from build123d import *

# Parameters (mm, degrees)
SKETCH1_R           = 4
BOSS_EXTRUDE1_DEPTH = 111
CUT_EXTRUDE1_START  = -0.8
SKETCH2_R           = 4
SKETCH2_R_2         = 3.75
CUT_EXTRUDE1_DEPTH  = 0.8
SKETCH4_R           = 4
BOSS_EXTRUDE3_DEPTH = 0.85
BOSS_EXTRUDE4_START = 0.8
SKETCH3_R           = 3.75
BOSS_EXTRUDE4_DEPTH = 0.8
BOSS_EXTRUDE5_START = 1
SKETCH5_R           = 4
BOSS_EXTRUDE5_DEPTH = 1
SKETCH6_W           = 3
SKETCH6_H           = 3
CUT_EXTRUDE2_DEPTH  = 20


with BuildPart() as part:
    # Sketch1 → Boss-Extrude1 (new body)
    with BuildSketch(Plane(origin=(0, 0, 0), x_dir=(1, 0, 0), z_dir=(0, 1, 0))):
        with Locations(Location((0, 0, 0), (0, 0, 270))):
            Circle(SKETCH1_R)
    extrude(amount=BOSS_EXTRUDE1_DEPTH)

    # Sketch2 → Cut-Extrude1 (cut)
    with BuildSketch(Plane(origin=(0, 86, 0), x_dir=(1, 0, 0), z_dir=(0, 1, 0)).offset(CUT_EXTRUDE1_START)):
        with Locations(Location((0, 0, 0), (0, 0, 270))):
            Circle(SKETCH2_R)
        with Locations(Location((0, 0, 0), (0, 0, 270))):
            Circle(SKETCH2_R_2, mode=Mode.SUBTRACT)
    extrude(amount=CUT_EXTRUDE1_DEPTH, mode=Mode.SUBTRACT)

    # Sketch4 → Boss-Extrude3 (add)
    with BuildSketch(Plane(origin=(0, 111, 0), x_dir=(1, 0, 0), z_dir=(0, 1, 0))):
        with Locations(Location((0, 0, 0), (0, 0, 270))):
            Circle(SKETCH4_R)
    extrude(amount=BOSS_EXTRUDE3_DEPTH)

    # Sketch3 → Boss-Extrude4 (add)
    with BuildSketch(Plane(origin=(0, 0, 0), x_dir=(-1, 0, 0), z_dir=(0, -1, 0)).offset(BOSS_EXTRUDE4_START)):
        with Locations(Location((0, 0, 0), (0, 0, 270))):
            Circle(SKETCH3_R)
    extrude(amount=-BOSS_EXTRUDE4_DEPTH)

    # Sketch5 → Boss-Extrude5 (add)
    with BuildSketch(Plane.XZ.offset(0.8).offset(BOSS_EXTRUDE5_START)):
        with Locations(Location((0, 0, 0), (0, 0, 90))):
            Circle(SKETCH5_R)
    extrude(amount=-BOSS_EXTRUDE5_DEPTH)

    # Sketch6 → Cut-Extrude2 (cut)
    with BuildSketch(Plane(origin=(0, 111.85, 0), x_dir=(1, 0, 0), z_dir=(0, 1, 0))):
        with Locations((0, 4)):
            Rectangle(SKETCH6_W, SKETCH6_H)
    extrude(amount=-CUT_EXTRUDE2_DEPTH, mode=Mode.SUBTRACT)


solid = part.part
Source: CAD feature listing. Evaluate the final solid. Frame: model axes, mm. A direction names the side the tool comes from. Give positions to 0.01 mm unless a question says otherwise; leave off trailing zeros. Write each loop counter-clockwise with the first axis right and the second up, starting at its lowest first coordinate (ties: lowest second). Pieces come first, ordered by that corner, then holes. Notation, with made-up numbers: M 20.5,-37.75 L 41.5,-37.75 A29 ccw 41.5,-4.75 Z; hole C -27,45 d11. An arc over 180 degrees is marked long. Return JSON: item names as keys, results as strings. Group by question number.
1) Draft query along Y for faces 4 (the face through (0, -1.8, 0)), 5 (the face through (0.165, 85.594, -3.746)), 6 (the face through (0, 111.85, 0)), 7 (the face through (3.905, -1.307, -0.867)). Return one class per face: released by +Y, released by -Y, zero draft, split by the parting line, or undercut.
2) Cut plane C-C, the plane z = -1.25. Output: boundary loops of the cut face in (x, y), then the cut area to 3 significant figures.
3) First-contact query: pin 1 Ø1.5 at (x, y) = (-0.5, 30.5) entering from -Z; pin 2 Ø1 at (y, z) = (104, -3.5) entering from -X; pin 3 Ø0.8 at (x, z) = (-0.5, -3) entering from +Y; pin 4 Ø3.5 at (x, y) = (0, 101.5) entering from -Z. Flat tips, straight axial feed; report the tip coordinate or a pass-through.
4) Ray query, L1, parallel to Y at x = 3, z = -2.5; L2, parallel to Z at x = 0.25, y = 78; L3, parallel to X at y = 77.5, z = -3.5. Return the intervals inside material, ascending.
5) Cut plane B-B, the plane y = 58. Output: boundary loops of the cut face in (x, z), then the cut area to 3 significant figures.
6) Set-up query: faces 1 (the face through (-0.165, -0.406, -3.746)), 2 (the face through (-3.905, 42.004, -0.867)), 3 (the face through (0, 102, -2.5)). Return all of +Z, -Z, +X, -X, +Y, -Y with unobstructed straight access to the full face (end or side cutting, diameter ignored); none if empty.
7) Cut plane A-A, the plane x = 0. Output: boundary loops of the cut face in (y, z), then the cut area to 3 significant figures.
Data:
{
 "1": {"face 4": "released by -Y", "face 5": "undercut", "face 6": "released by +Y", "face 7": "zero draft"},
 "2": {"outline": "M -3.8,-1.8 L 3.8,-1.8 L 3.8,-0.8 L 3.54,-0.8 L 3.54,0 L 3.8,0 L 3.8,85.2 L 3.54,85.2 L 3.54,86 L 3.8,86 L 3.8,111.85 L -3.8,111.85 L -3.8,86 L -3.54,86 L -3.54,85.2 L -3.8,85.2 L -3.8,0 L -3.54,0 L -3.54,-0.8 L -3.8,-0.8 Z", "area": "863 mm²"},
 "3": {"pin 1": "stops at z = -4", "pin 2": "stops at x = -2.65", "pin 3": "stops at y = 91.85", "pin 4": "stops at z = -3.71"},
 "4": {"L1": "y = -1.8 to -0.8, 0 to 85.2, 86 to 111.85", "L2": "z = -3.99 to 3.99", "L3": "x = -1.94 to 1.94"},
 "5": {"outline": "C 0,0 d8", "area": "50.3 mm²"},
 "6": {"face 1": "none", "face 2": "+Y, -Y", "face 3": "-Z, +Y"},
 "7": {"outline": "M -1.8,-4 L -0.8,-4 L -0.8,-3.75 L 0,-3.75 L 0,-4 L 85.2,-4 L 85.2,-3.75 L 86,-3.75 L 86,-4 L 91.85,-4 L 91.85,-2.5 L 111.85,-2.5 L 111.85,4 L 86,4 L 86,3.75 L 85.2,3.75 L 85.2,4 L 0,4 L 0,3.75 L -0.8,3.75 L -0.8,4 L -1.8,4 Z", "area": "878 mm²"}
}
